Geometry check sheet. Reference: the model listing, model coordinates, mm. Give positions to 0.01 mm unless a question says otherwise; leave off trailing zeros. Write each loop counter-clockwise with the first axis right and the second up, starting at its lowest first coordinate (ties: lowest second). Pieces come first, ordered by that corner, then holes. Notation, with made-up numbers: M 26,-9 L 45,-9 A23 cw 45,29 Z; hole C 24.5,82 d9. An arc over 180 degrees is marked long. Use one line per item in the form item = value. Start each with the question number.
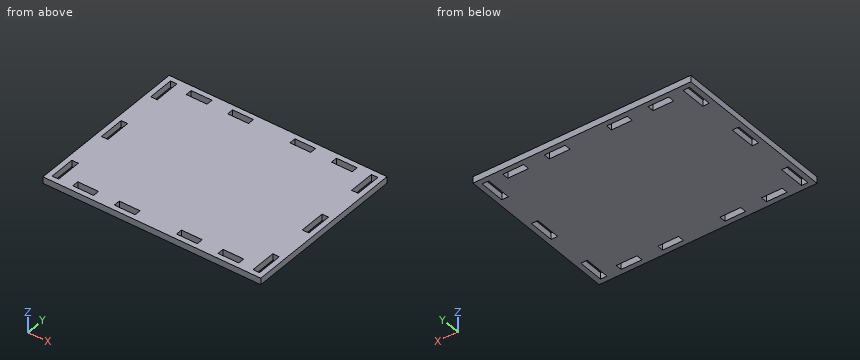
```python
from build123d import *

# Parameters (mm, degrees)
SKETCH1_W           = 84
SKETCH1_H           = 64
SKETCH1_W_2         = 8
SKETCH1_H_2         = 2.5
SKETCH1_W_3         = 2.5
SKETCH1_H_3         = 10
BOSS_EXTRUDE1_DEPTH = 2.5


with BuildPart() as part:
    # Sketch1 → Boss-Extrude1 (new body)
    with BuildSketch(Plane.XY):
        Rectangle(SKETCH1_W, SKETCH1_H)
        with Locations((-12, 28.75)):
            Rectangle(SKETCH1_W_2, SKETCH1_H_2, mode=Mode.SUBTRACT)
        with Locations((-28, 28.75)):
            Rectangle(SKETCH1_W_2, SKETCH1_H_2, mode=Mode.SUBTRACT)
        with Locations((-12, -28.75)):
            Rectangle(SKETCH1_W_2, SKETCH1_H_2, mode=Mode.SUBTRACT)
        with Locations((-28, -28.75)):
            Rectangle(SKETCH1_W_2, SKETCH1_H_2, mode=Mode.SUBTRACT)
        with Locations((-38.75, 0)):
            Rectangle(SKETCH1_W_3, SKETCH1_H_3, mode=Mode.SUBTRACT)
        with Locations((-38.75, 25)):
            Rectangle(SKETCH1_W_3, SKETCH1_H_3, mode=Mode.SUBTRACT)
        with Locations((-38.75, -25)):
            Rectangle(SKETCH1_W_3, SKETCH1_H_3, mode=Mode.SUBTRACT)
        with Locations((12, 28.75)):
            Rectangle(SKETCH1_W_2, SKETCH1_H_2, mode=Mode.SUBTRACT)
        with Locations((28, 28.75)):
            Rectangle(SKETCH1_W_2, SKETCH1_H_2, mode=Mode.SUBTRACT)
        with Locations((38.75, 25)):
            Rectangle(SKETCH1_W_3, SKETCH1_H_3, mode=Mode.SUBTRACT)
        with Locations((38.75, 0)):
            Rectangle(SKETCH1_W_3, SKETCH1_H_3, mode=Mode.SUBTRACT)
        with Locations((28, -28.75)):
            Rectangle(SKETCH1_W_2, SKETCH1_H_2, mode=Mode.SUBTRACT)
        with Locations((12, -28.75)):
            Rectangle(SKETCH1_W_2, SKETCH1_H_2, mode=Mode.SUBTRACT)
        with Locations((38.75, -25)):
            Rectangle(SKETCH1_W_3, SKETCH1_H_3, mode=Mode.SUBTRACT)
    extrude(amount=BOSS_EXTRUDE1_DEPTH)


solid = part.part
```
(1) Depth check by flat-ended pin: pin 1 (2 mm diameter, centred on x = -3.5, y = -14.5, fed in from -Z). Enter the tip coordinate at first touch or a pass-through.
(2) Sectioned sample at A-A, the plane x = -30. Record the boundary of the cut face in (y, z).
(3) Sectioned sample at C-C, the plane z = 0.6. State how many separate pieces and enclosed holes the cut face has, plus the area to 3 significant figures.
(4) Thickness scan on probe 1 along Y at (x, z) = (15, 0.55); probe 2 along X at (y, z) = (26, 0.8). Record the ranges inside material, lowest first. Write a range as [from, to].
(5) Sectioned sample at B-B, the plane y = 21. Record the boundary of the cut face in (x, z), plus the area to 4 significant figures.
Numbers:
q1.pin_1 = 0
q2.outline = M -32,0 L -30,0 L -30,2.5 L -32,2.5 Z; M -27.5,0 L 27.5,0 L 27.5,2.5 L -27.5,2.5 Z; M 30,0 L 32,0 L 32,2.5 L 30,2.5 Z
q3.separate_pieces = 1
q3.enclosed_holes = 14
q3.area = 5,070 mm2
q4.probe_1 = [-32, -30], [-27.5, 27.5], [30, 32]
q4.probe_2 = [-42, -40], [-37.5, 37.5], [40, 42]
q5.outline = M -42,0 L -40,0 L -40,2.5 L -42,2.5 Z; M -37.5,0 L 37.5,0 L 37.5,2.5 L -37.5,2.5 Z; M 40,0 L 42,0 L 42,2.5 L 40,2.5 Z
q5.area = 197.5 mm2
